Here's how the part is built. I have some questions about the finished solid (model axes, mm). A direction names the side the tool comes from. Coordinates: 2 decimals unless noted, no trailing zeros. Order: outer loops, then holes, each group sorted by start corner. A loop starts at its lowest first (then second) coordinate and runs counter-clockwise, first axis right, second up. Notation, with made-up numbers: (28.25, 69.5) - (77.25, 69.5) arc R17 cw to (77.25, 98.5) - close; hole circle Ø10 at (-33.75, 21.5). An arc over 180 degrees is marked (long way). Answer as CSV lines item,"result". Start each with the question number.
Item 1: We'd pull the mould along X, two halves only. Please class faces 4 (the face through (1, 0, 3.5)), 5 (the face through (0, 3, 0)), 6 (the face through (7, -2, -1)), 7 (the face through (4, -2, -1)): pulls with the +X half, pulls with the -X half, needs draft (parallel to the pull), parting line crosses it, or undercut.
Item 2: I'm going to push flat-ended pins straight in: pin 1 (1 mm diameter, centred on y = 2.5, z = 2, fed in from +X); pin 2 (1.5 mm diameter, centred on y = -2.5, z = -1.5, fed in from -X); pin 3 (1.5 mm diameter, centred on y = 3, z = -2.5, fed in from -X); pin 4 (4 mm diameter, centred on x = 2, z = -2.5, fed in from -Y). Where does each tip first touch, or does it pass through?
Item 3: Imagine slicing it at B-B on x = -1.75. List the corners of the cut face in (y, z) for me, and give its area (3 significant figures).
Item 4: Imagine slicing it at D-D on x = 5.25. List the corners of the cut face in (y, z) for me, and give its area (3 significant figures).
Item 5: On a 3-axis mill with a long thin cutter (end or side, diameter ignored), from which of +Z, -Z, +X, -X, +Y, -Y can I reach the whole of each face in a straight line? I mean faces 1 (the face through (3, 2, 0)), 2 (the face through (1.014, -3.045, -1.726)), 3 (the face through (-2, -0.1, -2.5)). Say none if no direction works.
Item 6: Imagine slicing it at C-C on z = 2.25. Count the separate pieces of the cut face and the enclosed holes in it, and give its area (3 significant figures).
Item 7: Imagine slicing it at A-A on y = 0. List the corners of the cut face in (x, z) for me.
Item 8: I need wall thicknesses on line 1 (Y direction, x = 2.5, z = 0); line 2 (X direction, y = 3, z = 1); line 3 (Y direction, x = -1, z = 0). Which ranges of each line are inside material? Lowest first, please.
from build123d import *

# Parameters (mm, degrees)
ESQUISSE5_OUTSIDE_W     = 15.98
ESQUISSE5_OUTSIDE_H     = 15.98
ENL_V_MAT_EXTRU_1_DEPTH = 2


with BuildPart() as part:
    # Esquisse4 → Révolution2 (revolve)
    with BuildSketch(Plane.XY, mode=Mode.PRIVATE) as r_volution2_sk:
        Polygon((10, 1.1), (10, 2), (7, 2.5), (7, 2), (4, 2.5), (4, 2), (2, 2), (2, 5), (0, 5), (0, 2.5), (-4, 2.5), (-4, 1.1), align=None)
    revolve(r_volution2_sk.sketch.rotate(Axis((0, 0, 0), (1, 0, 0)), 90), axis=Axis((0, 0, 0), (1, 0, 0)))

    # Esquisse5 outside → Enlèv. mat.-Extru.1 (cut)
    with BuildSketch(Plane(origin=(2, 0, 0), x_dir=(0, 0, -1), z_dir=(1, 0, 0))):
        Rectangle(ESQUISSE5_OUTSIDE_W, ESQUISSE5_OUTSIDE_H)
        Polygon((0, -4.041451884), (3.5, -2.020725942), (3.5, 2.020725942), (0, 4.041451884), (-3.5, 2.020725942), (-3.5, -2.020725942), align=None, mode=Mode.SUBTRACT)
    extrude(amount=-ENL_V_MAT_EXTRU_1_DEPTH, mode=Mode.SUBTRACT)


solid = part.part
Responses:
1,face 4,"needs draft"
1,face 5,"pulls with the -X half"
1,face 6,"undercut"
1,face 7,"undercut"
2,pin 1,"stops at x = 2"
2,pin 2,"stops at x = -4"
2,pin 3,"stops at x = 0"
2,pin 4,"stops at y = -3.75"
3,outline,"circle Ø5 at (0, 0); hole circle Ø2.2 at (0, 0)"
3,area,"15.8 mm^2"
4,outline,"circle Ø4.58 at (0, 0); hole circle Ø2.2 at (0, 0)"
4,area,"12.7 mm^2"
5,face 1,"none"
5,face 2,"-Z, +X, -X, -Y"
5,face 3,"-X"
6,separate pieces,"3"
6,enclosed holes,"0"
6,area,"24.0 mm^2"
7,outline,"(-4, -2.5) - (0, -2.5) - (0, -3.5) - (2, -3.5) - (2, -2) - (4, -2) - (4, -2.5) - (7, -2) - (7, -2.5) - (10, -2) - (10, -1.1) - (-4, -1.1) - close; (-4, 1.1) - (10, 1.1) - (10, 2) - (7, 2.5) - (7, 2) - (4, 2.5) - (4, 2) - (2, 2) - (2, 3.5) - (0, 3.5) - (0, 2.5) - (-4, 2.5) - close"
8,line 1,"y = -2 to -1.1, 1.1 to 2"
8,line 2,"x = 0 to 2"
8,line 3,"y = -2.5 to -1.1, 1.1 to 2.5"
